Here's how the part is built. I have some questions about the finished solid (model axes, mm). Face numbers are marked on the shaded views. Coordinates: 2 decimals unless noted, no trailing zeros. Write each loop counter-clockwise with the first axis right and the second up, starting at its lowest first coordinate (ties: lowest second). Pieces come first, ordered by that corner, then holes.
Solid Edge part; units mm, degrees
sketch "Sketch1" plane through (0, 0, 0) normal (0, 0, 1) x (1, 0, 0)
  line L0 (17, 0) -> (17, -23.2)
  arc A0 (17, -23.2) -> (16.7, -23.5) centre (16.7, -23.2) cw
  line L1 (16.7, -23.5) -> (0.3, -23.5)
  arc A1 (0.3, -23.5) -> (0, -23.2) centre (0.3, -23.2) cw
  line L2 (0, -23.2) -> (0, 0)
  line L3 (0, 0) -> (17, 0)
revolve "RevolvedProtrusion1" add sketch "Sketch1" angle 360 about axis through (0, 0, 0) along (1, 0, 0)
sketch "Sketch2" plane through (0, 0, 0) normal (0, 0, 1) x (1, 0, 0)
  line L0 (-2.5, 0) -> (-2.5, 20.05)
  line L1 (-2.5, 20.05) -> (3.6, 20.05)
  line L2 (3.6, 20.05) -> (3.6, 21)
  arc A0 (3.6, 21) -> (4.1, 21.5) centre (4.1, 21) cw
  line L3 (4.1, 21.5) -> (12.9, 21.5)
  arc A1 (12.9, 21.5) -> (13.4, 21) centre (12.9, 21) cw
  line L4 (13.4, 21) -> (13.4, 20.05)
  line L5 (13.4, 20.05) -> (19.5, 20.05)
  line L6 (19.5, 20.05) -> (19.5, 0)
  line L7 (19.5, 0) -> (-2.5, 0)
revolve "RevolvedCutout1" cut sketch "Sketch2" angle 360 about axis through (19.5, 0, 0) along (-1, 0, 0)
sketch "Sketch3" plane through (0, 0, 0) normal (0, 0, 1) x (1, 0, 0)
  circle A0 centre (8.5, 28.05) radius 5
revolve "RevolvedCutout2" cut sketch "Sketch3" angle 360 about axis through (13.5, 0, 0) along (-1, 0, 0)
sketch "Sketch4" plane through (0, 0, 0) normal (0, 0, 1) x (1, 0, 0)
  line L0 (15.6, 21.15) -> (15.6, 17.5)
  line L1 (15.6, 17.5) -> (17, 17.5)
  line L2 (17, 17.5) -> (17, 21.15)
  line L3 (17, 21.15) -> (15.6, 21.15)
revolve "RevolvedCutout3" cut sketch "Sketch4" angle 360 about axis through (55.5, 0, 0) along (-1, 0, 0)
sketch "Sketch5" plane through (0, 0, 0) normal (0, 0, 1) x (1, 0, 0)
  line L0 (0, 21.15) -> (0, 17.5)
  line L1 (0, 17.5) -> (1.4, 17.5)
  line L2 (1.4, 17.5) -> (1.4, 21.15)
  line L3 (1.4, 21.15) -> (0, 21.15)
revolve "RevolvedCutout4" cut sketch "Sketch5" angle 360 about axis through (55.5, 0, 0) along (-1, 0, 0)
sketch "Sketch6" plane through (0, 23.5, 0) normal (0, -1, 0) x (1, 0, 0)
  circle A0 centre (8.5, 0) radius 1.5
extrude "ExtrudedCutout_1" cut sketch "Sketch6" along normal blind 8
properties part number "NA 4906UU Outer ring" material "Aluminio, 7075-T6"
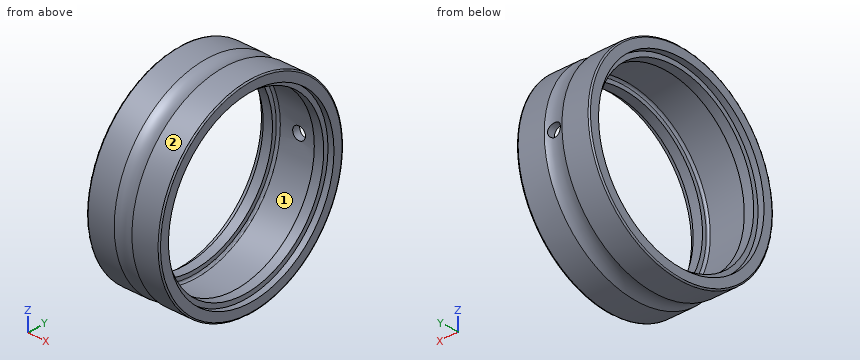
1) Imagine slicing it at C-C on x = 8.5. Please give me the cut outline in (y, z), then the cut area to 3 significant figures.
Values follow:
outline: (21.45, -1.5) arc R21.5 cw (long way) to (21.45, 1.5) - (23, 1.5) arc R23.05 ccw (long way) to (23, -1.5) - close
area: 212 mm2
2) Imagine slicing it at A-A on x = 5.5. Please give me the cut outline in (y, z).
Values follow:
outline: circle Ø47 at (0, 0); hole circle Ø43 at (0, 0)
3) Imagine slicing it at B-B on z = 0. Count the separate pieces of the cut face and the enclosed holes in it, then the cut area to 3 significant figures.
Values follow:
separate pieces: 3
enclosed holes: 0
area: 75.5 mm2
4) I need wall thicknesses on probe 1 along Y at (x, z) = (0.95, 0); probe 2 along X at (y, z) = (22, 0). Which ranges of each line are inside material? Lowest first, please.
Values follow:
probe 1: y = -23.5 to -21.15, 21.15 to 23.5
probe 2: x = 0 to 7, 10 to 17
5) Will these pins go through, and if not, where does the flat tip stop? pin 1 (6 mm diameter, centred on x = 13.5, y = -12, fed in from -Z); pin 2 (4 mm diameter, centred on x = 10, z = -12, fed in from +Y); pin 3 (10 mm diameter, centred on y = -11, z = -10.5, fed in from -X).
Values follow:
pin 1: stops at z = -21.71
pin 2: stops at y = 21.23
pin 3: stops at x = 1.4
6) We'd pull the mould along Z, two halves only. Please class the marked faces 1 and 2: pulls with the +Z half, pulls with the -Z half, needs draft (parallel to the pull), parting line crosses it, or undercut.
Values follow:
face 1: undercut
face 2: parting line crosses it
